Here's how the part is built. I have some questions about the finished solid (model axes, mm). A direction names the side the tool comes from. Coordinates: 2 decimals unless noted, no trailing zeros. Order: outer loops, then holes, each group sorted by start corner. A loop starts at its lowest first (then second) coordinate and runs counter-clockwise, first axis right, second up. Notation, with made-up numbers: (2.5, 75) - (46.5, 75) arc R23 ccw to (46.5, 110) - close; hole circle Ø2 at (-29, -14.5). An arc over 180 degrees is marked (long way). Answer in a Markdown table with one row per item. Add a question column.
Item 1: I want a section at B-B (x = 0.5). Please give me the cut outline in (y, z), plus the area to 3 significant figures.
Item 2: Thinking about a two-plate mould opening in X: for faces 4 (the cylindrical face through (0.525, -8.464, 4.056)), 5 (the flat face through (0, 4.5, 14)), 6 (the flat face through (4.15, 0, 6)), which applies, +X half, -X half, draft (parallel to the pull), parting line (faces both ways), or undercut?
Item 3: If I drill on line 1 along Y through (x, z) = (0.85, 3.25); line 2 along Z through (x, y) = (0, 0); line 3 along Z through (x, y) = (1.25, 12.25), over which ranges is the centre line in solid material (lowest first)? Write a range as from..to.
Item 4: I want a section at A-A (y = 7). Please give me the cut outline in (x, z).
Item 5: On a 3-axis mill with a long thin cutter (end or side, diameter ignored), from which of +Z, -Z, +X, -X, +Y, -Y can I reach the whole of each face in a straight line? I mean faces 1 (the flat face through (0, -4.5, 14)), 2 (the cylindrical face through (2.9, 0.06, 18.82)), 3 (the flat face through (0, 10, 8)). Say none if no direction works.
Item 6: I want a section at D-D (z = 4.5). Please give me the cut outline in (x, y), plus the area to 3 significant figures.
Item 7: Will these pins go through, and if not, where does the flat tip stop? pin 1 Ø3.5 at (x, y) = (0.85, -7) entering from +Z; pin 2 Ø1 at (x, y) = (1.5, 6.5) entering from +Z; pin 3 Ø2.5 at (x, z) = (0.5, 13.5) entering from +Y.
```python
from build123d import *

# Parameters (mm, degrees)
F0_W     = 8.3
F0_H     = 30
F1_DEPTH = 8
F2_R     = 1.5
F3_DEPTH = 8.001
F4_W     = 9
F4_H     = 12
F5_DEPTH = 8.3
F6_R     = 1.55
F7_DEPTH = 19.501
F8_R     = 4.14999


# Not quite as in the source:
# - a fillet or chamfer is up to 0.001 mm smaller than in the source, because OpenCascade refuses the exact size


with BuildPart() as f1:
    # F0 (on Top) → F1 (new body)
    with BuildSketch(Plane.XY):
        Rectangle(F0_W, F0_H)
    extrude(amount=F1_DEPTH)

    # F2 (on face) → F3 (cut, through all)
    with BuildSketch(Plane.XY.offset(8)):
        with Locations((0.85, -7)):
            Circle(F2_R)
        with Locations((0.85, 7)):
            Circle(F2_R)
    extrude(amount=-F3_DEPTH, mode=Mode.SUBTRACT)

    # F4 (on face) → F5 (join, through all)
    with BuildSketch(Plane.YZ.offset(4.15)):
        with Locations((0, 14)):
            Rectangle(F4_W, F4_H)
    extrude(amount=-F5_DEPTH)

    # F6 (on face) → F7 (cut, through all)
    with BuildSketch(Plane.XZ.offset(4.5)):
        with Locations((0, 15.85)):
            Circle(F6_R)
    extrude(amount=-F7_DEPTH, mode=Mode.SUBTRACT)

    # F8 (radius 4.15 in the source; OpenCascade refuses exactly that, so slightly less here)
    f8_edges = [f1.edges().sort_by_distance(p)[0] for p in [
        (4.15, 0, 20),
        (-4.15, 0, 20),
    ]]
    fillet(f8_edges, radius=F8_R)


solid = f1.part
```
Values follow:
| question | item | result |
|---|---|---|
| 1 | outline | (-15, 0) - (-8.46, 0) - (-8.46, 8) - (-15, 8) - close; (-5.54, 0) - (5.54, 0) - (5.54, 8) - (4.5, 8) - (4.5, 14.38) - (-4.5, 14.38) - (-4.5, 8) - (-5.54, 8) - close; (-4.5, 17.32) - (4.5, 17.32) - (4.5, 19.97) - (-4.5, 19.97) - close; (8.46, 0) - (15, 0) - (15, 8) - (8.46, 8) - close |
| 1 | area | 275 mm^2 |
| 2 | face 4 | undercut |
| 2 | face 5 | draft |
| 2 | face 6 | +X half |
| 3 | line 1 | y = -15..-8.5, -5.5..5.5, 8.5..15 |
| 3 | line 2 | z = 0..14.3, 17.4..20 |
| 3 | line 3 | z = 0..8 |
| 4 | outline | (-4.15, 0) - (-0.65, 0) - (-0.65, 8) - (-4.15, 8) - close; (2.35, 0) - (4.15, 0) - (4.15, 8) - (2.35, 8) - close |
| 5 | face 1 | +Z, +X, -X, -Y |
| 5 | face 2 | +Z, +X, +Y, -Y |
| 5 | face 3 | +Z, +X, -X, +Y |
| 6 | outline | (-4.15, -15) - (4.15, -15) - (4.15, 15) - (-4.15, 15) - close; hole circle Ø3 at (0.85, -7); hole circle Ø3 at (0.85, 7) |
| 6 | area | 235 mm^2 |
| 7 | pin 1 | stops at z = 8 |
| 7 | pin 2 | passes through |
| 7 | pin 3 | stops at y = 4.5 |
